from build123d import *

# Parameters (mm, degrees)
SKETCH1_W      = 16
SKETCH1_H      = 16
EXTRUDE1_DEPTH = 64
SKETCH2_W      = 13
SKETCH2_H      = 13
EXTRUDE2_DEPTH = 68.882250994
SKETCH3_R      = 4
SKETCH3_R_2    = 1.85
EXTRUDE3_DEPTH = 68.882250994
SKETCH4_R      = 4
SKETCH4_R_2    = 1.85
EXTRUDE4_DEPTH = 68.882250994
FILLET1_R      = 1


with BuildPart() as part:
    # Sketch1 → Extrude1 (new body)
    with BuildSketch(Plane.XY):
        with Locations((8, 8)):
            Rectangle(SKETCH1_W, SKETCH1_H)
    extrude(amount=-EXTRUDE1_DEPTH)

    # Sketch2 → Extrude2 (cut, through all)
    with BuildSketch(Plane.XY):
        with Locations((8, 8)):
            Rectangle(SKETCH2_W, SKETCH2_H)
    extrude(amount=-EXTRUDE2_DEPTH, mode=Mode.SUBTRACT)

    # Sketch3 → Extrude3 (cut, through all)
    with BuildSketch(Plane(origin=(0, 16, 0), x_dir=(1, 0, 0), z_dir=(0, 1, 0))):
        with Locations((8, 64)):
            Circle(SKETCH3_R)
        with Locations(Location((8, 32, 0), (0, 0, 270))):
            Circle(SKETCH3_R)
        with Locations((8, 0)):
            Circle(SKETCH3_R)
        with Locations((8, 96)):
            Circle(SKETCH3_R)
        with Locations((8, 128)):
            Circle(SKETCH3_R)
        with Locations((8, 160)):
            Circle(SKETCH3_R)
        with Locations((8, 192)):
            Circle(SKETCH3_R)
        with Locations((8, 224)):
            Circle(SKETCH3_R)
        with Locations((8, 256)):
            Circle(SKETCH3_R)
        with Locations(Location((8, 48, 0), (0, 0, 270))):
            Circle(SKETCH3_R)
        with Locations(Location((8, 56, 0), (0, 0, 270))):
            Circle(SKETCH3_R_2)
        with Locations(Location((8, 40, 0), (0, 0, 270))):
            Circle(SKETCH3_R_2)
        with Locations((8, 80)):
            Circle(SKETCH3_R)
        with Locations((8, 88)):
            Circle(SKETCH3_R_2)
        with Locations((8, 72)):
            Circle(SKETCH3_R_2)
        with Locations(Location((8, 16, 0), (0, 0, 270))):
            Circle(SKETCH3_R)
        with Locations(Location((8, 24, 0), (0, 0, 270))):
            Circle(SKETCH3_R_2)
        with Locations(Location((8, 8, 0), (0, 0, 270))):
            Circle(SKETCH3_R_2)
        with Locations((8, 112)):
            Circle(SKETCH3_R)
        with Locations((8, 120)):
            Circle(SKETCH3_R_2)
        with Locations((8, 104)):
            Circle(SKETCH3_R_2)
        with Locations((8, 144)):
            Circle(SKETCH3_R)
        with Locations((8, 152)):
            Circle(SKETCH3_R_2)
        with Locations((8, 136)):
            Circle(SKETCH3_R_2)
        with Locations((8, 176)):
            Circle(SKETCH3_R)
        with Locations((8, 184)):
            Circle(SKETCH3_R_2)
        with Locations((8, 168)):
            Circle(SKETCH3_R_2)
        with Locations((8, 208)):
            Circle(SKETCH3_R)
        with Locations((8, 216)):
            Circle(SKETCH3_R_2)
        with Locations((8, 200)):
            Circle(SKETCH3_R_2)
        with Locations((8, 240)):
            Circle(SKETCH3_R)
        with Locations((8, 248)):
            Circle(SKETCH3_R_2)
        with Locations((8, 232)):
            Circle(SKETCH3_R_2)
    extrude(amount=-EXTRUDE3_DEPTH, mode=Mode.SUBTRACT)

    # Sketch4 → Extrude4 (cut, through all)
    with BuildSketch(Plane(origin=(16, 0, 0), x_dir=(0, 0, -1), z_dir=(1, 0, 0))):
        with Locations(Location((32, 8, 0), (0, 0, 90))):
            Circle(SKETCH4_R)
        with Locations((64, 8)):
            Circle(SKETCH4_R)
        with Locations((0, 8)):
            Circle(SKETCH4_R)
        with Locations((96, 8)):
            Circle(SKETCH4_R)
        with Locations((128, 8)):
            Circle(SKETCH4_R)
        with Locations((160, 8)):
            Circle(SKETCH4_R)
        with Locations((192, 8)):
            Circle(SKETCH4_R)
        with Locations((224, 8)):
            Circle(SKETCH4_R)
        with Locations((256, 8)):
            Circle(SKETCH4_R)
        with Locations(Location((48, 8.074203, 0), (0, 0, 90))):
            Circle(SKETCH4_R)
        with Locations(Location((40, 8.074203, 0), (0, 0, 90))):
            Circle(SKETCH4_R_2)
        with Locations(Location((56, 8.074203, 0), (0, 0, 90))):
            Circle(SKETCH4_R_2)
        with Locations((80, 8)):
            Circle(SKETCH4_R)
        with Locations((72, 8)):
            Circle(SKETCH4_R_2)
        with Locations((88, 8)):
            Circle(SKETCH4_R_2)
        with Locations(Location((16, 8, 0), (0, 0, 90))):
            Circle(SKETCH4_R)
        with Locations(Location((8, 8, 0), (0, 0, 90))):
            Circle(SKETCH4_R_2)
        with Locations(Location((24, 8, 0), (0, 0, 90))):
            Circle(SKETCH4_R_2)
        with Locations((112, 8)):
            Circle(SKETCH4_R)
        with Locations((104, 8)):
            Circle(SKETCH4_R_2)
        with Locations((120, 8)):
            Circle(SKETCH4_R_2)
        with Locations((144, 8)):
            Circle(SKETCH4_R)
        with Locations((136, 8)):
            Circle(SKETCH4_R_2)
        with Locations((152, 8)):
            Circle(SKETCH4_R_2)
        with Locations((176, 8)):
            Circle(SKETCH4_R)
        with Locations((168, 8)):
            Circle(SKETCH4_R_2)
        with Locations((184, 8)):
            Circle(SKETCH4_R_2)
        with Locations((208, 8)):
            Circle(SKETCH4_R)
        with Locations((200, 8)):
            Circle(SKETCH4_R_2)
        with Locations((216, 8)):
            Circle(SKETCH4_R_2)
        with Locations((240, 8)):
            Circle(SKETCH4_R)
        with Locations((232, 8)):
            Circle(SKETCH4_R_2)
        with Locations((248, 8)):
            Circle(SKETCH4_R_2)
    extrude(amount=-EXTRUDE4_DEPTH, mode=Mode.SUBTRACT)

    # Fillet1
    fillet1_edges = [part.edges().sort_by_distance(p)[0] for p in [
        (0, 16, -32),
        (16, 16, -32),
        (16, 0, -32),
        (0, 0, -32),
    ]]
    fillet(fillet1_edges, radius=FILLET1_R)


solid = part.part
Source: CAD feature listing. Evaluate the final solid. Frame: model axes, mm. Give positions to 0.01 mm unless a question says otherwise; leave off trailing zeros. Write each loop counter-clockwise with the first axis right and the second up, starting at its lowest first coordinate (ties: lowest second). Pieces come first, ordered by that corner, then holes. Notation, with made-up numbers: M 84,5 L 134,5 A7 cw 134,17 Z; hole C 21,59 d4. An arc over 180 degrees is marked long. Return JSON: item names as keys, results as strings. Group by question number.
1) Draft query along X for faces 1 (the face through (14.5, 3.6, -31.6)), 2 (the face through (8, 15, -4)), 3 (the face through (1, 14, 0)). Return one class per face: released by +X, released by -X, zero draft, split by the parting line, or undercut.
2) First-contact query: pin 1 Ø5 at (x, z) = (8, -56) entering from -Y; pin 2 Ø2 at (x, y) = (1.5, 10) entering from -Z. Flat tips, straight axial feed; report the tip coordinate or a pass-through.
3) Ray query, L1, parallel to X at y = 11.5, z = -54.5; L2, parallel to X at y = 14.9, z = -8. Return the intervals inside material, ascending.
4) Cut plane A-A, the plane z = -16. Output: boundary loops of the cut face in (x, y).
5) Cut plane D-D, the plane z = -8. Output: boundary loops of the cut face in (x, y), then the cut area to 3 significant figures.
6) Cut plane B-B, the plane y = 3. Output: boundary loops of the cut face in (x, z).
Data:
{
 "1": {"face 1": "undercut", "face 2": "undercut", "face 3": "zero draft"},
 "2": {"pin 1": "stops at y = 0", "pin 2": "stops at z = -61.35"},
 "3": {"L1": "x = 0 to 1.5, 14.5 to 16", "L2": "x = 0 to 6.15, 9.85 to 16"},
 "4": {"outline": "M 0,1 A1 ccw 1,0 L 4,0 L 4,1.5 L 1.5,1.5 L 1.5,4 L 0,4 Z; M 0,12 L 1.5,12 L 1.5,14.5 L 4,14.5 L 4,16 L 1,16 A1 ccw 0,15 Z; M 12,0 L 15,0 A1 ccw 16,1 L 16,4 L 14.5,4 L 14.5,1.5 L 12,1.5 Z; M 12,14.5 L 14.5,14.5 L 14.5,12 L 16,12 L 16,15 A1 ccw 15,16 L 12,16 Z"},
 "5": {"outline": "M 0,1 A1 ccw 1,0 L 6.15,0 L 6.15,1.5 L 1.5,1.5 L 1.5,6.15 L 0,6.15 Z; M 0,9.85 L 1.5,9.85 L 1.5,14.5 L 6.15,14.5 L 6.15,16 L 1,16 A1 ccw 0,15 Z; M 9.85,0 L 15,0 A1 ccw 16,1 L 16,6.15 L 14.5,6.15 L 14.5,1.5 L 9.85,1.5 Z; M 9.85,14.5 L 14.5,14.5 L 14.5,9.85 L 16,9.85 L 16,15 A1 ccw 15,16 L 9.85,16 Z", "area": "63.9 mm²"},
 "6": {"outline": "M 0,-64 L 1.5,-64 L 1.5,0 L 0,0 Z; M 14.5,-64 L 16,-64 L 16,0 L 14.5,0 Z"}
}
